Could you check a few things on this model? Use its own coordinates, in mm. A direction names the side the tool comes from. Give positions to 0.01 mm unless a question says otherwise; leave off trailing zeros. Order: outer loops, then holes, each group sorted by start corner. A loop starts at its lowest first (then second) coordinate and runs counter-clockwise, first axis right, second up.
(1) On a 3-axis mill with a long thin cutter (end or side, diameter ignored), from which of +Z, -Z, +X, -X, +Y, -Y can I reach the whole of each face in a straight line? I mean faces 5 (the flat face through (18, -25, 4)), 6 (the flat face through (15, -31, 2)), 7 (the cylindrical face through (34.489, 19.515, 3.944)), 8 (the flat face through (-17.9, 29, 2)), 9 (the cylindrical face through (-2.4, 23.93, 4.06)). Say none if no direction works.
(2) If I drill on probe 1 along X at (y, z) = (23, 1.25) (3 decimals); probe 2 along Y at (x, z) = (-31, 4.5); probe 3 along Y at (x, z) = (-5, 4.5), over which ranges is the centre line in solid material (lowest first)?
(3) Imagine slicing it at B-B, the plane x = -9.5. Write out the boundary of the cut face in (y, z), then the cut area to 3 significant figures.
(4) Imagine slicing it at A-A, the plane x = 24. Write out the boundary of the cut face in (y, z), then the cut area to 3 significant figures.
(5) If we mould it in two halves opening along X, with no side actions, what happens to faces 1 (the flat face through (-11.1, -29, 2)), 2 (the cylindrical face through (-34.489, -19.515, 3.944)), 3 (the cylindrical face through (-2.4, -20.57, 4.06)), 4 (the flat face through (0, 0, 0))? For each: released by +X, released by -X, zero draft, split by the parting line, or undercut.
(6) Will these pins go through, and if not, where does the flat tip stop? pin 1 (3 mm diameter, centred on x = -4.5, z = 3.5, fed in from +Y); pin 2 (1.5 mm diameter, centred on x = -19.5, y = 8.5, fed in from -Z); pin 3 (3 mm diameter, centred on y = -30, z = 3, fed in from -X); pin 4 (2.5 mm diameter, centred on x = 26, z = 5, fed in from -Y).
Solid Edge part; units mm, degrees
sketch "Sketch1" plane through (0, 0, 0) normal (0, 0, 1) x (1, 0, 0)
  line L0 (-18, -27.5) -> (18, -27.5)
  line L1 (18, -27.5) -> (18, -21.7)
  arc A0 (18, -21.7) -> (19.7, -20) centre (19.7, -21.7) cw
  line L2 (19.7, -20) -> (33.3, -20)
  arc A1 (33.3, -20) -> (35, -18.3) centre (33.3, -18.3) ccw
  line L3 (35, -18.3) -> (35, 18.3)
  arc A2 (33.3, 20) -> (35, 18.3) centre (33.3, 18.3) cw
  line L4 (33.3, 20) -> (19.7, 20)
  arc A3 (18, 21.7) -> (19.7, 20) centre (19.7, 21.7) ccw
  line L5 (18, 21.7) -> (18, 27.5)
  line L6 (18, 27.5) -> (-18, 27.5)
  line L7 (-18, 27.5) -> (-18, 21.7)
  arc A4 (-19.7, 20) -> (-18, 21.7) centre (-19.7, 21.7) ccw
  line L8 (-19.7, 20) -> (-33.3, 20)
  arc A5 (-35, 18.3) -> (-33.3, 20) centre (-33.3, 18.3) cw
  line L9 (-35, 18.3) -> (-35, -18.3)
  arc A6 (-35, -18.3) -> (-33.3, -20) centre (-33.3, -18.3) ccw
  line L10 (-33.3, -20) -> (-19.7, -20)
  arc A7 (-19.7, -20) -> (-18, -21.7) centre (-19.7, -21.7) cw
  line L11 (-18, -21.7) -> (-18, -27.5)
extrude "Protrusion1" add sketch "Sketch1" along normal blind 8
sketch "Sketch2" plane through (0, -27.5, 4) normal (0, -1, 0) x (1, 0, 0)
  line L0 (-11.1, 0.8) -> (-17.9, 0.8)
  line L1 (-17.9, 0.8) -> (-17.9, -4)
  line L2 (-17.9, -4) -> (-11.1, -4)
  line L3 (-11.1, -4) -> (-11.1, 0.8)
  line L4 (11.1, 0.8) -> (17.9, 0.8)
  line L5 (17.9, 0.8) -> (17.9, -4)
  line L6 (17.9, -4) -> (11.1, -4)
  line L7 (11.1, -4) -> (11.1, 0.8)
extrude "ExtrudedProtrusion_2" add sketch "Sketch2" along normal blind 3.5
sketch "Sketch3" plane through (0, 27.5, 4) normal (0, 1, 0) x (-1, 0, 0)
  line L0 (-17.9, 0.8) -> (-11.1, 0.8)
  line L1 (-11.1, 0.8) -> (-11.1, -4)
  line L2 (-11.1, -4) -> (-17.9, -4)
  line L3 (-17.9, -4) -> (-17.9, 0.8)
extrude "ExtrudedProtrusion_3" add sketch "Sketch3" along normal blind 3.5
sketch "Sketch4" plane through (0, 0, 0) normal (0, 0, -1) x (0, 1, 0)
  arc A0 (-27.5, -8) -> (-27.5, -11) centre (-27.5, -9.5) cw
  line L0 (-27.5, -8) -> (-27.5, -11)
  arc A1 (-27.5, 11) -> (-27.5, 8) centre (-27.5, 9.5) cw
  line L1 (-27.5, 8) -> (-27.5, 11)
  arc A2 (27.5, -11) -> (27.5, -8) centre (27.5, -9.5) cw
  line L2 (27.5, -8) -> (27.5, -11)
  arc A3 (27.5, 8) -> (27.5, 11) centre (27.5, 9.5) cw
  line L3 (27.5, 8) -> (27.5, 11)
extrude "ExtrudedCutout_2" cut sketch "Sketch4" against normal blind 8
sketch "Sketch5" plane through (0, 27.5, 4) normal (0, 1, 0) x (-1, 0, 0)
  line L0 (11.1, 0.8) -> (17.9, 0.8)
  line L1 (17.9, 0.8) -> (17.9, -4)
  line L2 (17.9, -4) -> (11.1, -4)
  line L3 (11.1, -4) -> (11.1, 0.8)
extrude "ExtrudedProtrusion_4" add sketch "Sketch5" along normal blind 3.5
sketch "Sketch6" plane through (0, 0, 8) normal (0, 0, 1) x (-1, 0, 0)
  arc A0 (-1.5998, 20.0476) -> (1.5998, 20.0476) centre (0, 20.0254) ccw
  arc A1 (2.725, 21.5) -> (1.5998, 20.0476) centre (1.225, 21.5) cw
  line L0 (2.725, 23) -> (2.725, 21.5)
  arc A2 (1.5998, 24.4524) -> (2.725, 23) centre (1.225, 23) cw
  line L1 (1.5998, 27.5) -> (1.5998, 24.4524)
  line L2 (0, 27.5) -> (1.5998, 27.5)
  line L3 (0, 27.5) -> (-1.6, 27.5)
  line L4 (-1.6, 27.5) -> (-1.6, 24.4524)
  arc A3 (-1.6, 24.4524) -> (-2.725, 23) centre (-1.225, 23) ccw
  line L5 (-2.725, 23) -> (-2.725, 21.5)
  arc A4 (-2.725, 21.5) -> (-1.5998, 20.0476) centre (-1.225, 21.5) ccw
  arc A5 (-1.5998, -20.0476) -> (1.5998, -20.0476) centre (0, -20.0254) cw
  arc A6 (2.725, -21.5) -> (1.5998, -20.0476) centre (1.225, -21.5) ccw
  line L6 (2.725, -23) -> (2.725, -21.5)
  arc A7 (1.5998, -24.4524) -> (2.725, -23) centre (1.225, -23) ccw
  line L7 (1.5998, -27.5) -> (1.5998, -24.4524)
  line L8 (0, -27.5) -> (1.5998, -27.5)
  line L9 (0, -27.5) -> (-1.6, -27.5)
  line L10 (-1.6, -27.5) -> (-1.6, -24.4524)
  arc A8 (-1.6, -24.4524) -> (-2.725, -23) centre (-1.225, -23) cw
  line L11 (-2.725, -23) -> (-2.725, -21.5)
  arc A9 (-2.725, -21.5) -> (-1.5998, -20.0476) centre (-1.225, -21.5) cw
extrude "Cutout1" cut sketch "Sketch6" against normal up to next
properties material "Polycarbonate"
Answer block:
1. face 5: +Z, -Z, +X, -Y
1. face 6: +Z, -Z, +X, -X, -Y
1. face 7: +Z, -Z, +X, +Y
1. face 8: +Z, -Z, -X, +Y
1. face 9: +Z, -Z
2. probe 1: x = -18 to -2.725, 2.725 to 18
2. probe 2: y = -20 to 20
2. probe 3: y = -27.5 to 27.5
3. outline: (-26, 0) - (26, 0) - (26, 8) - (-26, 8) - close
3. area: 416 mm2
4. outline: (-20, 0) - (20, 0) - (20, 8) - (-20, 8) - close
4. area: 320 mm2
5. face 1: undercut
5. face 2: released by -X
5. face 3: undercut
5. face 4: zero draft
6. pin 1: stops at y = 27.5
6. pin 2: stops at z = 0
6. pin 3: stops at x = -17.9
6. pin 4: stops at y = -20
